Build history of the part. All positions in model axes, mm. A direction names the side the tool comes from. Round coordinates to 2 decimals unless told otherwise and drop trailing zeros. Write each loop counter-clockwise with the first axis right and the second up, starting at its lowest first coordinate (ties: lowest second). Pieces come first, ordered by that corner, then holes. Notation, with made-up numbers: (32, 82) -> (44, 82) arc R13 cw to (44, 105) -> close; hole circle Ø10 at (-14, 8.5). An arc over 180 degrees is marked (long way). Answer in a Markdown table with one row per item. Add a question column.
from build123d import *

# Parameters (mm, degrees)
F0_W         = 12
F0_H         = 3.2
F1_DEPTH     = 20
F3_D         = 5.5
F4_W         = 18.2
F4_H         = 1.6
F5_DEPTH     = 0.9
F6_T1_DEPTH  = 18.2
F6_T6_DEPTH  = 18.2
F6_T11_DEPTH = 18.2
F6_T16_DEPTH = 18.2
F6_T21_DEPTH = 18.2
F6_T26_DEPTH = 18.2
F6_T31_DEPTH = 18.2
F6_T36_DEPTH = 18.2
F7_R         = 5


# Not quite as in the source:
# - a fillet or chamfer that OpenCascade refuses, or shapes differently, is made with other operations: its cross-section is extruded or revolved along the edge and cut away or added


with BuildPart() as f1:
    # F0 (on Front) → F1 (new body)
    with BuildSketch(Plane.XZ):
        Polygon((-9.1, 10.5), (0, 10.5), (0, 12.9), (-11.5, 12.9), (-11.5, 3.2), (-11.5, 0), (-9.1, 0), align=None)
        with Locations((-17.5, 1.6)):
            Rectangle(F0_W, F0_H)
        Polygon((0, 12.9), (0, 10.5), (9.1, 10.5), (9.1, 0), (11.5, 0), (11.5, 3.2), (11.5, 12.9), align=None)
        with Locations((17.5, 1.6)):
            Rectangle(F0_W, F0_H)
    extrude(amount=F1_DEPTH)

    # F3 (through all)
    with Locations(Plane.XY.offset(3.2)):
        with Locations((-17.5, -10), (17.5, -10)):
            Hole(F3_D / 2)

    # F4 (on face) → F5 (join)
    with BuildSketch(Plane(origin=(0, 0, 10.5), x_dir=(1, 0, 0), z_dir=(0, 0, -1))):
        with Locations((0, 0.8)):
            Rectangle(F4_W, F4_H)
        with Locations((0, 4)):
            Rectangle(F4_W, F4_H)
        with Locations((0, 7.2)):
            Rectangle(F4_W, F4_H)
        with Locations((0, 10.4)):
            Rectangle(F4_W, F4_H)
    extrude(amount=F5_DEPTH)

    # F6: chamfer of 1 on 8 edges, made by hand

    # F6_s2 → F6_t1 (cut)
    with BuildSketch(Plane.YZ.offset(-9.1)):
        Polygon((-1, 9.6), (0, 10.6), (0, 9.6), align=None)
    extrude(amount=F6_T1_DEPTH, mode=Mode.SUBTRACT)


with BuildPart() as f6_tool4:
    # F6_s5 → F6_t6 (new body)
    with BuildSketch(Plane.YZ.offset(9.1)):
        Polygon((-1.6, 10.6), (-0.6, 9.6), (-1.6, 9.6), align=None)
    extrude(amount=-F6_T6_DEPTH)

    split(bisect_by=Plane.XY.offset(10.5), keep=Keep.BOTTOM)


with BuildPart() as f1_1:
    add(f1.part)

    # F6_t3: cut F6_tool4
    add(f6_tool4.part, mode=Mode.SUBTRACT)


with BuildPart() as f6_tool9:
    # F6_s10 → F6_t11 (new body)
    with BuildSketch(Plane.YZ.offset(-9.1)):
        Polygon((-3.2, 10.6), (-4.2, 9.6), (-3.2, 9.6), align=None)
    extrude(amount=F6_T11_DEPTH)

    split(bisect_by=Plane.XY.offset(10.5), keep=Keep.BOTTOM)


with BuildPart() as f1_2:
    add(f1_1.part)

    # F6_t8: cut F6_tool9
    add(f6_tool9.part, mode=Mode.SUBTRACT)


with BuildPart() as f6_tool14:
    # F6_s15 → F6_t16 (new body)
    with BuildSketch(Plane.YZ.offset(9.1)):
        Polygon((-4.8, 10.6), (-3.8, 9.6), (-4.8, 9.6), align=None)
    extrude(amount=-F6_T16_DEPTH)

    split(bisect_by=Plane.XY.offset(10.5), keep=Keep.BOTTOM)


with BuildPart() as f1_3:
    add(f1_2.part)

    # F6_t13: cut F6_tool14
    add(f6_tool14.part, mode=Mode.SUBTRACT)


with BuildPart() as f6_tool19:
    # F6_s20 → F6_t21 (new body)
    with BuildSketch(Plane.YZ.offset(-9.1)):
        Polygon((-7.4, 9.6), (-6.4, 10.6), (-6.4, 9.6), align=None)
    extrude(amount=F6_T21_DEPTH)

    split(bisect_by=Plane.XY.offset(10.5), keep=Keep.BOTTOM)


with BuildPart() as f1_4:
    add(f1_3.part)

    # F6_t18: cut F6_tool19
    add(f6_tool19.part, mode=Mode.SUBTRACT)


with BuildPart() as f6_tool24:
    # F6_s25 → F6_t26 (new body)
    with BuildSketch(Plane.YZ.offset(9.1)):
        Polygon((-8, 10.6), (-7, 9.6), (-8, 9.6), align=None)
    extrude(amount=-F6_T26_DEPTH)

    split(bisect_by=Plane.XY.offset(10.5), keep=Keep.BOTTOM)


with BuildPart() as f1_5:
    add(f1_4.part)

    # F6_t23: cut F6_tool24
    add(f6_tool24.part, mode=Mode.SUBTRACT)


with BuildPart() as f6_tool29:
    # F6_s30 → F6_t31 (new body)
    with BuildSketch(Plane.YZ.offset(-9.1)):
        Polygon((-10.6, 9.6), (-9.6, 10.6), (-9.6, 9.6), align=None)
    extrude(amount=F6_T31_DEPTH)

    split(bisect_by=Plane.XY.offset(10.5), keep=Keep.BOTTOM)


with BuildPart() as f1_6:
    add(f1_5.part)

    # F6_t28: cut F6_tool29
    add(f6_tool29.part, mode=Mode.SUBTRACT)


with BuildPart() as f6_tool34:
    # F6_s35 → F6_t36 (new body)
    with BuildSketch(Plane.YZ.offset(9.1)):
        Polygon((-11.2, 10.6), (-10.2, 9.6), (-11.2, 9.6), align=None)
    extrude(amount=-F6_T36_DEPTH)

    split(bisect_by=Plane.XY.offset(10.5), keep=Keep.BOTTOM)


with BuildPart() as f1_7:
    add(f1_6.part)

    # F6_t33: cut F6_tool34
    add(f6_tool34.part, mode=Mode.SUBTRACT)

    # F7
    f7_edges = [f1_7.edges().sort_by_distance(p)[0] for p in [
        (-23.5, -20, 1.6),
        (23.5, -20, 1.6),
        (23.5, 0, 1.6),
        (-23.5, 0, 1.6),
    ]]
    fillet(f7_edges, radius=F7_R)


solid = f1_7.part
(1) Which spindle directions (+Z, -Z, +X, -X, +Y, -Y) get a long thin tool onto all of the face, cutting with end or side? Do faces 1 (the face through (-15, -12, 3.2)), 2 (the face through (11.5, -10, 8)), 3 (the face through (0, -15, 10.5)). Say none if no direction does.
(2) Saw through at B-B (z = 7). List the corners of the cut face in (x, y).
(3) Drop flat-ended pins along their axis: P1, Ø5, axis at y = -11.5, z = 8, coming from the -X side; P2, Ø9.5, axis at x = 18, y = -9.5, coming from the +Z side; P3, Ø1.4, axis at x = 1, y = -8.5, coming from the -Z side. Give the stop position or say it passes through.
(4) Mould opens along Y. For faces 4 (the face through (0, -6, 10.5)), 5 (the face through (-22.07, -18.5, 1.62)), 6 (the face through (-0.1, -0.4, 10.2)) say: pulls with the +Y half, pulls with the -Y half, needs draft (parallel to the pull), parting line crosses it, or undercut.
(5) Probe line 1 along X through (y, z) = (-9.75, 1.25); line 2 along Y through (x, z) = (17.5, 1.05); line 3 along X through (y, z) = (-4, 4.5). List the from-to ranges inside material, lowest first.
(6) Saw through at D-D (x = 3). List the corners of the cut face in (y, z), plus the area to 3 significant figures.
(7) Saw through at A-A (x = -17.5). List the corners of the cut face in (y, z), plus the area to 3 significant figures.
(8) Saw through at C-C (y = -12.25). List the corners of the cut face in (x, z).
Answer sheet:
| question | item | result |
|---|---|---|
| 1 | face 1 | +Z, -X, +Y, -Y |
| 1 | face 2 | +Z, +X, +Y, -Y |
| 1 | face 3 | -Z, -Y |
| 2 | outline | (-11.5, -20) -> (-9.1, -20) -> (-9.1, 0) -> (-11.5, 0) -> close; (9.1, -20) -> (11.5, -20) -> (11.5, 0) -> (9.1, 0) -> close |
| 3 | P1 | stops at x = -11.5 |
| 3 | P2 | stops at z = 3.2 |
| 3 | P3 | stops at z = 10.4 |
| 4 | face 4 | undercut |
| 4 | face 5 | pulls with the -Y half |
| 4 | face 6 | pulls with the +Y half |
| 5 | line 1 | x = -23.5 to -20.24, -14.76 to -9.1, 9.1 to 14.76, 20.24 to 23.5 |
| 5 | line 2 | y = -20 to -12.75, -7.25 to 0 |
| 5 | line 3 | x = -11.5 to -9.1, 9.1 to 11.5 |
| 6 | outline | (-20, 10.5) -> (-11.1, 10.5) -> (-10.4, 9.8) -> (-9.7, 10.5) -> (-7.9, 10.5) -> (-7.2, 9.8) -> (-6.5, 10.5) -> (-4.7, 10.5) -> (-4, 9.8) -> (-3.3, 10.5) -> (-1.5, 10.5) -> (-0.8, 9.8) -> (0, 10.6) -> (0, 12.9) -> (-20, 12.9) -> close |
| 6 | area | 50.0 mm² |
| 7 | outline | (-20, 0) -> (-12.75, 0) -> (-12.75, 3.2) -> (-20, 3.2) -> close; (-7.25, 0) -> (0, 0) -> (0, 3.2) -> (-7.25, 3.2) -> close |
| 7 | area | 46.4 mm² |
| 8 | outline | (-23.5, 0) -> (-19.08, 0) -> (-19.08, 3.2) -> (-23.5, 3.2) -> close; (-15.92, 0) -> (-9.1, 0) -> (-9.1, 10.5) -> (9.1, 10.5) -> (9.1, 0) -> (15.92, 0) -> (15.92, 3.2) -> (11.5, 3.2) -> (11.5, 12.9) -> (-11.5, 12.9) -> (-11.5, 3.2) -> (-15.92, 3.2) -> close; (19.08, 0) -> (23.5, 0) -> (23.5, 3.2) -> (19.08, 3.2) -> close |
